Here's how the part is built. I have some questions about the finished solid (model axes, mm). Coordinates: 2 decimals unless noted, no trailing zeros. Loops run counter-clockwise (first coordinate to the right, second up) from the corner with the lowest first, then second, coordinate; pieces in that order, holes last. Notation, with made-up numbers: (64.5, 63.25) - (104.5, 63.25) arc R20 cw to (104.5, 91.25) - close; hole circle Ø8 at (88, -6). An arc over 180 degrees is marked (long way). Use a Markdown table: item, result.
```python
from build123d import *

# Parameters (mm, degrees)
SKETCH2_W                                       = 50
SKETCH2_H                                       = 10
BOSS_EXTRUDE1_DEPTH                             = 50
TAP_DRILL_FOR_M10_TAP1_D                        = 8.5
CSK_FOR_M5_FLAT_HEAD_MACHINE_SCREW2_D           = 5.5
CSK_FOR_M5_FLAT_HEAD_MACHINE_SCREW2_CSINK_D     = 10.4
CSK_FOR_M5_FLAT_HEAD_MACHINE_SCREW2_CSINK_ANGLE = 90


with BuildPart() as part:
    # Sketch2 → Boss-Extrude1 (new body)
    with BuildSketch(Plane.XY):
        with Locations((25, 5)):
            Rectangle(SKETCH2_W, SKETCH2_H)
    extrude(amount=BOSS_EXTRUDE1_DEPTH)

    # Tap Drill for M10 Tap1 (through all)
    with Locations(Plane(origin=(0, 10, 0), x_dir=(1, 0, 0), z_dir=(0, 1, 0))):
        with Locations((17.5, -25), (32.5, -25)):
            Hole(TAP_DRILL_FOR_M10_TAP1_D / 2)

    # CSK for M5 Flat Head Machine Screw2 (through all)
    with Locations(Plane(origin=(0, 10, 0), x_dir=(1, 0, 0), z_dir=(0, 1, 0))):
        with Locations((7.5, -7.5), (42.5, -7.5), (42.5, -42.5), (7.5, -42.5)):
            CounterSinkHole(CSK_FOR_M5_FLAT_HEAD_MACHINE_SCREW2_D / 2, CSK_FOR_M5_FLAT_HEAD_MACHINE_SCREW2_CSINK_D / 2, counter_sink_angle=CSK_FOR_M5_FLAT_HEAD_MACHINE_SCREW2_CSINK_ANGLE)


solid = part.part
```
Q1. If we mould it in two halves opening along X, with no side actions, what happens to faces 1 (the face through (25, 5, 0)), 2 (the face through (0, 5, 25)), 3 (the face through (7.858, 3.722, 39.773))? For each: pulls with the +X half, pulls with the -X half, needs draft (parallel to the pull), parting line crosses it, or undercut.
Check values:
| item | result |
|---|---|
| face 1 | needs draft |
| face 2 | pulls with the -X half |
| face 3 | undercut |
Q2. I want a section at D-D, the plane x = 21. Write out the boundary of the cut face in (y, z), then the cut area to 3 significant figures.
Check values:
| item | result |
|---|---|
| outline | (0, 0) - (10, 0) - (10, 22.59) - (0, 22.59) - close; (0, 27.41) - (10, 27.41) - (10, 50) - (0, 50) - close |
| area | 452 mm^2 |
Q3. Please list where these lines run through material, in increasing order: L1, parallel to Z at x = 42.5, y = 5; L2, parallel to X at y = 6.5, z = 25. Write a range as from..to.
Check values:
| item | result |
|---|---|
| L1 | 0..4.75, 10.25..39.75, 45.25..50 |
| L2 | 0..13.25, 21.75..28.25, 36.75..50 |
Q4. I want a section at A-A, the plane z = 25. Write out the boundary of the cut face in (x, y), then the cut area to 3 significant figures.
Check values:
| item | result |
|---|---|
| outline | (0, 0) - (13.25, 0) - (13.25, 10) - (0, 10) - close; (21.75, 0) - (28.25, 0) - (28.25, 10) - (21.75, 10) - close; (36.75, 0) - (50, 0) - (50, 10) - (36.75, 10) - close |
| area | 330 mm^2 |
Q5. I want a section at C-C, the plane y = 3. Write out the boundary of the cut face in (x, z), then the cut area to 3 significant figures.
Check values:
| item | result |
|---|---|
| outline | (0, 0) - (50, 0) - (50, 50) - (0, 50) - close; hole circle Ø5.5 at (7.5, 7.5); hole circle Ø5.5 at (7.5, 42.5); hole circle Ø8.5 at (17.5, 25); hole circle Ø8.5 at (32.5, 25); hole circle Ø5.5 at (42.5, 7.5); hole circle Ø5.5 at (42.5, 42.5) |
| area | 2,290 mm^2 |
Q6. I want a section at B-B, the plane x = 42.5. Write out the boundary of the cut face in (y, z), then the cut area to 3 significant figures.
Check values:
| item | result |
|---|---|
| outline | (0, 0) - (10, 0) - (10, 2.3) - (7.55, 4.75) - (0, 4.75) - close; (0, 10.25) - (7.55, 10.25) - (10, 12.7) - (10, 37.3) - (7.55, 39.75) - (0, 39.75) - close; (0, 45.25) - (7.55, 45.25) - (10, 47.7) - (10, 50) - (0, 50) - close |
| area | 378 mm^2 |
Q7. Will these pins go through, and if not, where does the flat tip stop? P1, Ø7, axis at x = 7.5, z = 7.5, coming from the +Y side; P2, Ø6.5, axis at x = 42.5, z = 7.5, coming from the +Y side.
Check values:
| item | result |
|---|---|
| P1 | y = 8.3 |
| P2 | y = 8.05 |
